Can you work these out from the model? Positions are in its coordinate system, mm. Face numbers are marked on the shaded views. A direction names the side the tool comes from. Round coordinates to 2 decimals unless told otherwise and drop trailing zeros. Order: outer loops, then holes, each group sorted by start corner. A loop starts at its lowest first (then second) coordinate and runs counter-clockwise, first axis right, second up. Notation, with made-up numbers: M -11,64 L 27,64 A10 ccw 27,72 Z; hole C -28,41.25 d6. An arc over 180 degrees is marked long. One line per question, with ' | ' between items.
```python
from build123d import *

# Parameters (mm, degrees)
F0_W     = 0.0066861176
F0_H     = 1.2904889882
F0_W_2   = 32.9669154744
F0_W_3   = 0.0352981806
F1_DEPTH = 12.7


with BuildPart() as f1:
    # F0 (on Front) → F1 (new body)
    with BuildSketch(Plane.XZ):
        with Locations((-3.0995408706, -47.3976228386)):
            Rectangle(F0_W, F0_H)
        Polygon((-8.27790464, -48.0428673327), (-3.1028839294, -48.0428673327), (-3.1028839294, -46.7523783445), (-3.0961978118, -46.7523783445), (-3.0961978118, -37.0955993858), (3.972609491, -37.0955993858), (3.972609491, -32.1745417944), (-3.0961978118, -32.1745417944), (-3.0961978118, -0.1459635726), (-8.8304810221, -0.1459635726), (-31.4444088096, -32.3726352144), (-31.4444088096, -37.0955993858), (-8.27790464, -37.0955993858), align=None)
        with BuildLine():
            Line((-8.27790464, -16.3374941646), (-8.27790464, -32.1745417944))
            Line((-8.27790464, -32.1745417944), (-26.033330653, -32.1745417944))
            Line((-26.033330653, -32.1745417944), (-11.1450462452, -10.9993977943))
            add(Edge.make_bspline(
                [(-8.2049228537, -5.8176909661), (-9.7688182747, -8.945481808), (-11.1450462452, -10.9993977943)],
                knots=[0, 0, 0, 1, 1, 1], degree=2))
            Line((-8.2049228537, -5.8176909661), (-7.9442736169, -5.8176909661))
            add(Edge.make_bspline(
                [(-8.27790464, -16.3374941646), (-8.27790464, -11.67708581), (-7.9442736169, -5.8176909661)],
                knots=[0, 0, 0, 1, 1, 1], degree=2))
        make_face(mode=Mode.SUBTRACT)
        with Locations((13.3872599254, -47.3976228386)):
            Rectangle(F0_W_2, F0_H)
        with Locations((29.8883667529, -47.3976228386)):
            Rectangle(F0_W_3, F0_H)
        Polygon((29.9060158432, -46.7523783445), (29.9060158432, -48.0428673327), (35.0524244908, -48.0428673327), (35.0524244908, -37.0955993858), (42.1212317936, -37.0955993858), (42.1212317936, -32.1745417944), (35.0524244908, -32.1745417944), (35.0524244908, -0.1459635726), (29.3181412805, -0.1459635726), (6.704213493, -32.3726352144), (6.704213493, -37.0955993858), (29.8707176626, -37.0955993858), (29.8707176626, -46.7523783445), align=None)
        with BuildLine():
            Line((29.8707176626, -16.3374941646), (29.8707176626, -32.1745417944))
            Line((29.8707176626, -32.1745417944), (12.1152916496, -32.1745417944))
            Line((12.1152916496, -32.1745417944), (27.0035760574, -10.9993977943))
            add(Edge.make_bspline(
                [(29.9436994489, -5.8176909661), (28.3798040279, -8.945481808), (27.0035760574, -10.9993977943)],
                knots=[0, 0, 0, 1, 1, 1], degree=2))
            Line((29.9436994489, -5.8176909661), (30.2043486857, -5.8176909661))
            add(Edge.make_bspline(
                [(29.8707176626, -16.3374941646), (29.8707176626, -11.67708581), (30.2043486857, -5.8176909661)],
                knots=[0, 0, 0, 1, 1, 1], degree=2))
        make_face(mode=Mode.SUBTRACT)
    extrude(amount=F1_DEPTH)


solid = f1.part
```
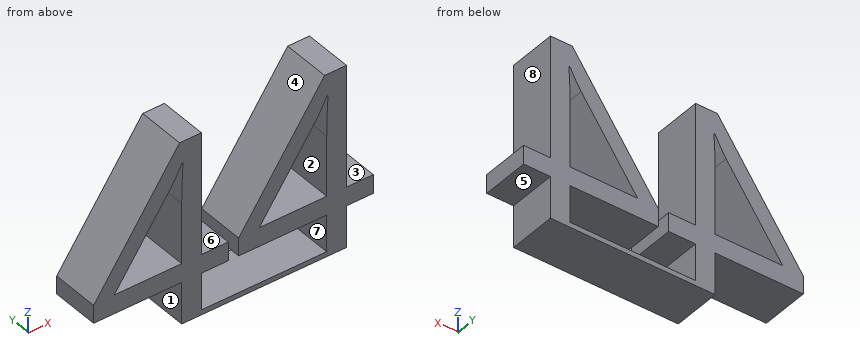
(1) If we section it at B-B on x = 14: Please give me the cut outline in (y, z), plus the area to 3 significant figures.
Final values:
outline: M -12.7,-48.04 L 0,-48.04 L 0,-46.75 L -12.7,-46.75 Z; M -12.7,-37.1 L 0,-37.1 L 0,-32.17 L -12.7,-32.17 Z; M -12.7,-29.49 L 0,-29.49 L 0,-21.98 L -12.7,-21.98 Z | area: 174 mm^2
(2) If we section it at A-A on z = -35: Please give me the cut outline in (x, y).
Final values:
outline: M -31.44,-12.7 L 3.97,-12.7 L 3.97,0 L -31.44,0 Z; M 6.7,-12.7 L 42.12,-12.7 L 42.12,0 L 6.7,0 Z
(3) On a 3-axis mill with a long thin cutter (end or side, diameter ignored), from which of +Z, -Z, +X, -X, +Y, -Y can I reach the whole of each face in a straight line? I mean the marked faces 1, 2, 3, 4 and 5. Say none if no direction works.
Final values:
face 1: -Z, -X, +Y, -Y | face 2: +Y, -Y | face 3: +Z, +X, +Y, -Y | face 4: +Z, +Y, -Y | face 5: -Z, +X, +Y, -Y
(4) Thinking about a two-plate mould opening in Z: for the marked faces 6, 7 and 8, which applies, released by +Z, released by -Z, zero draft, split by the parting line, or undercut?
Final values:
face 6: released by +Z | face 7: undercut | face 8: zero draft
(5) If we section it at D-D on z = -40.5: Please give me the cut outline in (x, y), plus the area to 3 significant figures.
Final values:
outline: M -8.28,-12.7 L -3.1,-12.7 L -3.1,0 L -8.28,0 Z; M 29.87,-12.7 L 35.05,-12.7 L 35.05,0 L 29.87,0 Z | area: 132 mm^2
(6) Will these pins go through, and if not, where does the flat tip stop? pin 1 Ø4 at (y, z) = (-5.5, -22.5) entering from +X; pin 2 Ø3 at (y, z) = (-5, -41.5) entering from -X; pin 3 Ø3.5 at (x, y) = (39, -5) entering from -Z.
Final values:
pin 1: x = 35.05 | pin 2: x = -8.28 | pin 3: z = -37.1
(7) Please list where these lines run through material, in increasing order: probe 1 along X at (y, z) = (-2.5, -12); probe 2 along X at (y, z) = (-9.75, -24); probe 3 along Z at (x, y) = (14.5, -1). Write a range as [from, to].
Final values:
probe 1: [-17.15, -11.85], [-8.21, -3.1], [21, 26.3], [29.94, 35.05] | probe 2: [-25.57, -20.29], [-8.28, -3.1], [12.58, 17.86], [29.87, 35.05] | probe 3: [-48.04, -46.75], [-37.1, -32.17], [-28.78, -21.26]
(8) If we section it at C-C on z = -28: Please give me the cut outline in (x, y).
Final values:
outline: M -28.38,-12.7 L -23.1,-12.7 L -23.1,0 L -28.38,0 Z; M -8.28,-12.7 L -3.1,-12.7 L -3.1,0 L -8.28,0 Z; M 9.77,-12.7 L 15.05,-12.7 L 15.05,0 L 9.77,0 Z; M 29.87,-12.7 L 35.05,-12.7 L 35.05,0 L 29.87,0 Z
